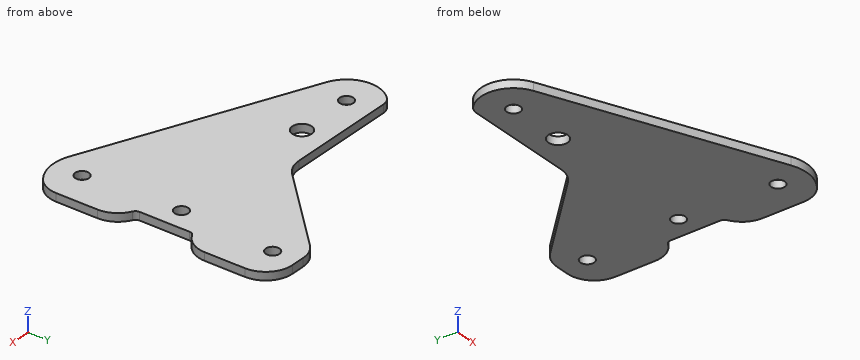
```python
from build123d import *

# Parameters (mm, degrees)
SKETCH1_R           = 2.55
SKETCH1_R_2         = 3.6
BOSS_EXTRUDE1_DEPTH = 3


with BuildPart() as part:
    # Sketch1 → Boss-Extrude1 (new body)
    with BuildSketch(Plane.XY):
        with BuildLine():
            Line((-40.320217865, 38.096664926), (0.519782135, 38.096664926))
            ThreePointArc((0.519782135, 38.096664926), (4.346616459, 38.857869601), (7.590849947, 41.025597114))
            Line((7.590849947, 41.025597114), (36.7307204, 70.165467567))
            ThreePointArc((36.7307204, 70.165467567), (39.974953888, 72.33319508), (43.801788211, 73.094399755))
            Line((43.801788211, 73.094399755), (48.931788211, 73.094399755))
            ThreePointArc((48.931788211, 73.094399755), (56.002856023, 70.165467567), (58.931788211, 63.094399755))
            Line((58.931788211, 63.094399755), (58.931788211, 48.094399755))
            ThreePointArc((58.931788211, 48.094399755), (57.46359146, 42.87823897), (53.490121545, 39.193748249))
            ThreePointArc((53.490121545, 39.193748249), (52.695427562, 38.456850105), (52.401788211, 37.413617948))
            Line((52.401788211, 37.413617948), (52.401788211, 18.773617948))
            ThreePointArc((52.401788211, 18.773617948), (52.695427562, 17.730385791), (53.490121545, 16.993487647))
            ThreePointArc((53.490121545, 16.993487647), (57.46359146, 13.308996927), (58.931788211, 8.092836142))
            Line((58.931788211, 8.092836142), (58.931788211, -7.287163858))
            ThreePointArc((58.931788211, -7.287163858), (57.846780817, -11.817385358), (54.827206843, -15.364542093))
            ThreePointArc((54.827206843, -15.364542093), (47.694417569, -18.15064712), (40.115883144, -17.052976855))
            Line((40.115883144, -17.052976855), (-40.115883144, 17.052976855))
            ThreePointArc((-40.115883144, 17.052976855), (-47.212985277, 25.870194867), (-43.819425953, 36.668155197))
            ThreePointArc((-43.819425953, 36.668155197), (-42.209999419, 37.725782086), (-40.320217865, 38.096664926))
        make_face()
        with Locations((-35.421326542, 28.096578546)):
            Circle(SKETCH1_R, mode=Mode.SUBTRACT)
        with Locations((-13.931326542, 28.096578546)):
            Circle(SKETCH1_R_2, mode=Mode.SUBTRACT)
        with Locations((46.221788211, 63.594399755)):
            Circle(SKETCH1_R, mode=Mode.SUBTRACT)
        with Locations((44.271788211, 28.094399755)):
            Circle(SKETCH1_R, mode=Mode.SUBTRACT)
        with Locations((46.264570837, -7.409030505)):
            Circle(SKETCH1_R, mode=Mode.SUBTRACT)
    extrude(amount=BOSS_EXTRUDE1_DEPTH)


solid = part.part
```
Design review of the part built by this model. Coordinates are the model's own, in mm. Give positions to 0.01 mm unless a question says otherwise; leave off trailing zeros. Loops run counter-clockwise (first coordinate to the right, second up) from the corner with the lowest first, then second, coordinate; pieces in that order, holes last. Notation, with made-up numbers: M 32,85 L 40,85 A21 cw 40,112 Z; hole C 16.5,54.25 d4. An arc over 180 degrees is marked long. Return JSON: item names as keys, results as strings. Group by question number.
Item 1: We need section D-D (x = 38.5). Give the boundary of the cut face in (y, z).
Item 2: We need section B-B (z = 0.7). Give the boundary of the cut face in (x, y), and give its area (3 significant figures).
Item 3: We need section A-A (x = -16). Give the boundary of the cut face in (y, z).
Item 4: We need section C-C (y = 1). Give the boundary of the cut face in (x, z).
Item 5: For probe 1 along X at (y, z) = (29, 1.95); probe 2 along Y at (x, z) = (-16.5, 0.25); probe 3 along Y at (x, z) = (-11, 2), list the stretches that pass through material, from the lowest coordinate up.
Item 6: Insertion check: pin 1 Ø6 at (x, y) = (-13.93, 28.1) entering from +Z; pin 2 Ø0.9 at (y, z) = (30.5, 2) entering from +X; pin 3 Ø1.5 at (y, z) = (-2.5, 2) entering from -X. Each pin has a flat end and moves straight along its axis. Give the tip position at first contact, or say it passes through.
Output:
{
 "1": {"outline": "M -16.37,0 L 71.57,0 L 71.57,3 L -16.37,3 Z"},
 "2": {"outline": "M -43.82,36.67 A12 ccw -40.12,17.05 L 40.12,-17.05 A15 ccw 54.83,-15.36 A10 ccw 58.93,-7.29 L 58.93,8.09 A10 ccw 53.49,16.99 A2 cw 52.4,18.77 L 52.4,37.41 A2 cw 53.49,39.19 A10 ccw 58.93,48.09 L 58.93,63.09 A10 ccw 48.93,73.09 L 43.8,73.09 A10 ccw 36.73,70.17 L 7.59,41.03 A10 cw 0.52,38.1 L -40.32,38.1 A5 ccw Z; hole C -35.42,28.1 d5.1; hole C -13.93,28.1 d7.2; hole C 44.27,28.09 d5.1; hole C 46.22,63.59 d5.1; hole C 46.26,-7.41 d5.1", "area": "5,170 mm^2"},
 "3": {"outline": "M 6.8,0 L 25.15,0 L 25.15,3 L 6.8,3 Z; M 31.04,0 L 38.1,0 L 38.1,3 L 31.04,3 Z"},
 "4": {"outline": "M -2.35,0 L 58.93,0 L 58.93,3 L -2.35,3 Z"},
 "5": {"probe 1": "x = -47.39 to -37.81, -33.04 to -17.42, -10.45 to 41.89, 46.66 to 52.4", "probe 2": "y = 7.01 to 25.57, 30.62 to 38.1", "probe 3": "y = 4.68 to 26.01, 30.19 to 38.1"},
 "6": {"pin 1": "passes through", "pin 2": "stops at x = 52.4", "pin 3": "stops at x = 4.12"}
}
